For this review, use the dimensioned drawing (mm, ordinates from the lowest corner) and the shaded views. A direction names the side the tool comes from. Round coordinates to 2 decimals unless told otherwise and drop trailing zeros. Write each loop counter-clockwise with the first axis right and the second up, starting at its lowest first coordinate (ties: lowest second). Pieces come first, ordered by that corner, then holes. Notation, with made-up numbers: M 1.5,68.5 L 27.5,68.5 A29 cw 27.5,88.5 Z; hole C 87,-33 d2. An arc over 180 degrees is marked long. Use one line per item in the form item = value. Start each with the question number.
Item 1: For line 1 (X direction, y = 0.25, z = 3.7); line 2 (Z direction, x = 3.75, y = 2.9); line 3 (Y direction, x = 1, z = 2.15), list the stretches that pass through material, from the lowest coordinate up. Write a range as [from, to].
Item 2: Draft analysis for pull direction Y (two halves, no side actions). For the marked faces 3, 4 and 5, state which applies: released by +Y, released by -Y, zero draft, split by the parting line, or undercut.
Item 3: Add section A-A (y = 2.7). State the section outline as (x, z) points.
Item 4: Add section C-C (z = 3.55). State the section outline as (x, y) points.
Item 5: For P1, Ø0.5, axis at y = 2.5, z = 1.5, coming from the -X side; P2, Ø1.4, axis at x = 5.5, z = 2.5, coming from the +Y side, all flat-tipped, find the tip position at first contact; note any pin that passes through.
Item 6: Add section D-D (z = 4.6). State the section outline as (x, y) points.
Item 7: Add section B-B (x = 9). State the section outline as (y, z) points, and give its area (3 significant figures).
Item 8: For the marked faces 1 and 2, list the 3-axis set-ups (+Z, -Z, +X, -X, +Y, -Y) from which the entire face can be reached by the end or side of a thin tool; tool diameter is ignored.
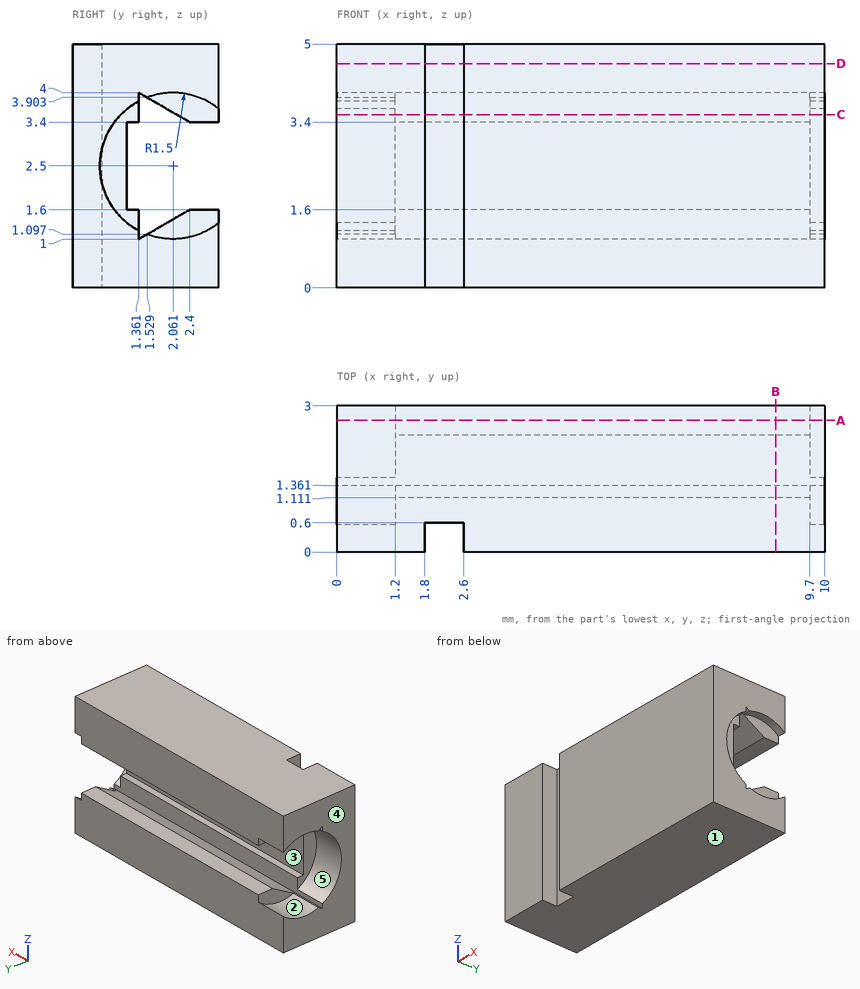
Calculated:
q1.line_1 = [0, 1.8], [2.6, 10]
q1.line_2 = [0, 1.6], [3.4, 5]
q1.line_3 = [0, 0.6]
q2.face_3 = released by +Y
q2.face_4 = zero draft
q2.face_5 = undercut
q3.outline = M 0,0 L 10,0 L 10,1.14 L 9.7,1.14 L 9.7,1.6 L 1.2,1.6 L 1.2,1.14 L 0,1.14 Z; M 0,3.86 L 1.2,3.86 L 1.2,3.4 L 9.7,3.4 L 9.7,3.86 L 10,3.86 L 10,5 L 0,5 Z
q4.outline = M 0,0 L 1.8,0 L 1.8,0.6 L 2.6,0.6 L 2.6,0 L 10,0 L 10,0.99 L 9.7,0.99 L 9.7,1.36 L 1.2,1.36 L 1.2,0.99 L 0,0.99 Z; M 1.2,2.14 L 9.7,2.14 L 9.7,3 L 1.2,3 Z
q5.P1 = 1.2
q5.P2 = 1.11
q6.outline = M 0,0 L 1.8,0 L 1.8,0.6 L 2.6,0.6 L 2.6,0 L 10,0 L 10,3 L 0,3 Z
q7.outline = M 0,0 L 3,0 L 3,1.6 L 2.4,1.6 L 1.36,1 L 1.36,1.6 L 1.11,1.6 L 1.11,3.4 L 1.36,3.4 L 1.36,4 L 2.4,3.4 L 3,3.4 L 3,5 L 0,5 Z
q7.area = 11.0 mm^2
q8.face_1 = -Z, +X, -X, +Y, -Y
q8.face_2 = -X
